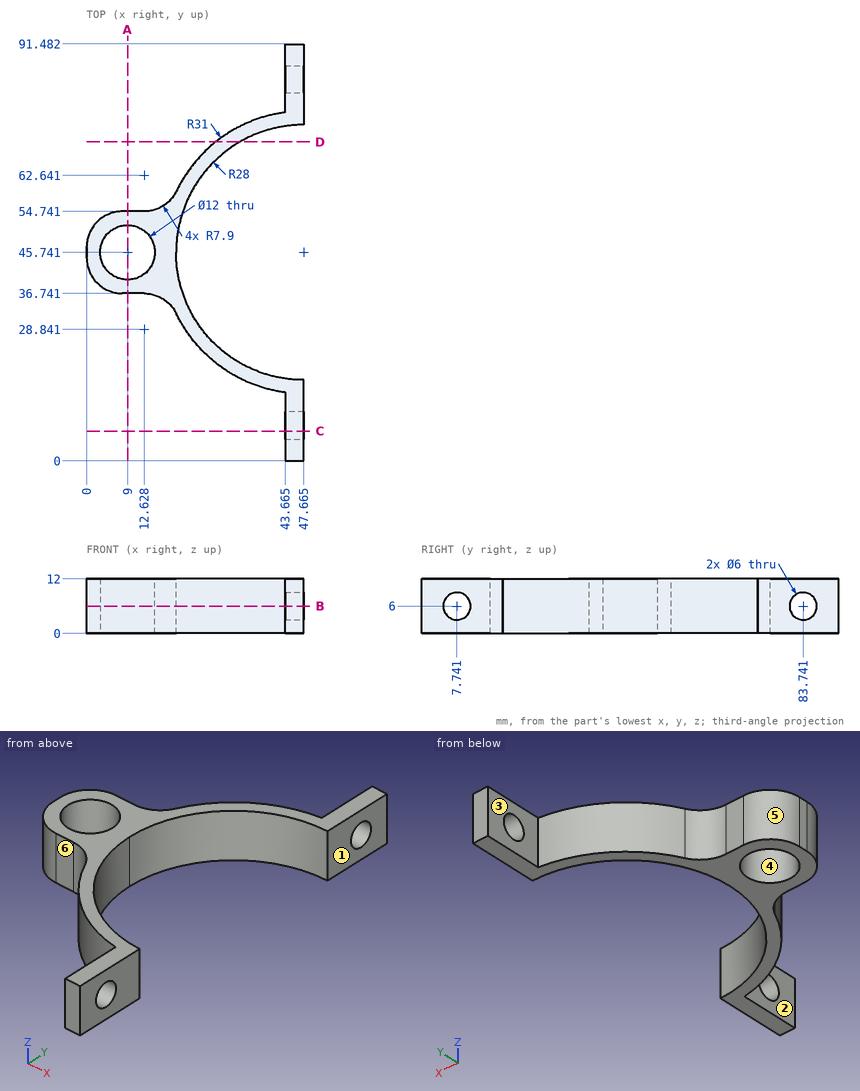
Design review of the part shown in the three views and the two pictorial views. Dimensions are in mm from the part's minimum x, y and z. A direction names the side the tool comes from. Coordinates: 2 decimals unless noted, no trailing zeros. Write each loop counter-clockwise with the first axis right and the second up, starting at its lowest first coordinate (ties: lowest second). Pieces come first, ordered by that corner, then holes. Notation, with made-up numbers: (13, -1) - (21, -1) arc R18 cw to (21, 31) - close; hole circle Ø3 at (61.25, 65). An arc over 180 degrees is marked (long way). Write item = value, one per line.
(1) Machinability: for the marked faces 1, 2 and 3, which of the approach directions +Z, -Z, +X, -X, +Y, -Y give a long, thin tool a straight path to every point of the face, cutting with its end or side? Answer none if there is none.
Result sheet:
face_1 = +Z, -Z, +X, +Y, -Y
face_2 = +Z, -Z, -X, -Y
face_3 = +Z, -Z, -X, +Y
(2) Consider section B-B, the plane z = 6. Give the boundary of the cut face in (x, y) (1 decimal).
Result sheet:
outline = (0, 44.6) arc R7.9 ccw to (7.9, 36.7) - (12.6, 36.7) arc R7.9 cw to (19.7, 32.3) arc R31 ccw to (43.7, 15) - (43.7, 10.7) - (47.7, 10.7) - (47.7, 17.7) arc R28 cw to (47.7, 73.7) - (47.7, 80.7) - (43.7, 80.7) - (43.7, 76.5) arc R31 ccw to (19.7, 59.2) arc R7.9 cw to (12.6, 54.7) - (7.9, 54.7) arc R7.9 ccw to (0, 46.8) - close; (43.7, 0) - (47.7, 0) - (47.7, 4.7) - (43.7, 4.7) - close; (43.7, 86.7) - (47.7, 86.7) - (47.7, 91.5) - (43.7, 91.5) - close; hole circle Ø12 at (9, 45.7)
(3) Consider section C-C, the plane y = 6.5. Give the boundary of the cut face in (x, z) (1 decimal).
Result sheet:
outline = (43.7, 0) - (47.7, 0) - (47.7, 3.3) - (43.7, 3.3) - close; (43.7, 8.7) - (47.7, 8.7) - (47.7, 12) - (43.7, 12) - close
(4) For line 1 (Y direction, x = 9, z = 6.75); line 2 (X direction, y = 7, z = 10.5) (1 decimal); line 3 (Y direction, x = 8, z = 10.5) (1 decimal), list the stretches that pass through material, from the lowest coordinate up. Write a range as [from, to].
Result sheet:
line_1 = [36.74, 39.74], [51.74, 54.74]
line_2 = [43.7, 47.7]
line_3 = [36.7, 39.8], [51.7, 54.7]
(5) Consider section D-D, the plane y = 70. Give the boundary of the cut face in (x, z) (1 decimal), then the cut area to 3 significant figures.
Result sheet:
outline = (28.4, 0) - (33.7, 0) - (33.7, 12) - (28.4, 12) - close
area = 63.8 mm^2
(6) Consider section A-A, the plane x = 9. Give the boundary of the cut face in (y, z).
Result sheet:
outline = (36.74, 0) - (39.74, 0) - (39.74, 12) - (36.74, 12) - close; (51.74, 0) - (54.74, 0) - (54.74, 12) - (51.74, 12) - close
(7) For P1, Ø3.5, axis at y = 87.5, z = 8.5, coming from the -X side (1 decimal); P2, Ø5, axis at x = 10.5, z = 8, coming from the -Y side; P3, Ø19, axis at x = 9, y = 45.74, coming from the -Z side; P4, Ø4, axis at x = 10.5, z = 4, coming from the +Y side, all flat-tipped, find the tip position at first contact; note any pin that passes through.
Result sheet:
P1 = 43.7
P2 = 36.73
P3 = 0
P4 = 54.74
(8) Mouldability with a two-part tool opening along X and no side actions: class the marked faces 4, 5 and 6 as pulls with the +X half, pulls with the -X half, needs draft (parallel to the pull), parting line crosses it, or undercut.
Result sheet:
face_4 = undercut
face_5 = pulls with the -X half
face_6 = needs draft
